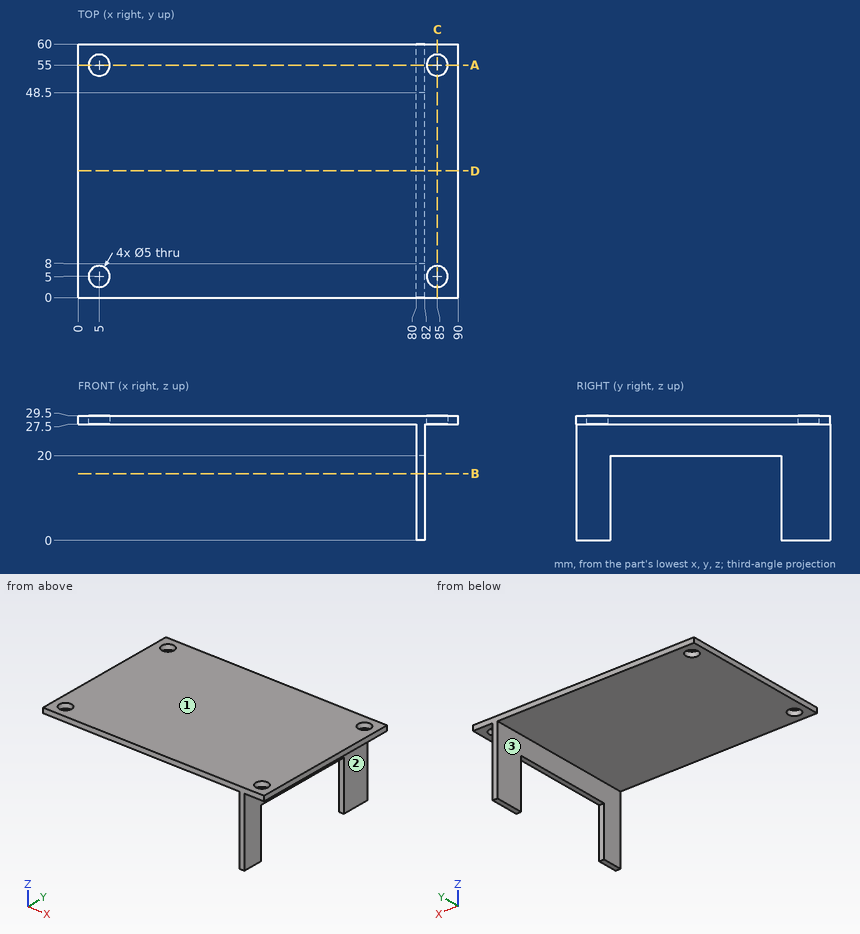
Could you check a few things on this drawing? It's one solid part, dimensions in mm from its lowest x, y, z. A direction names the side the tool comes from. Round coordinates to 2 decimals unless told otherwise and drop trailing zeros. Write each loop counter-clockwise with the first axis right and the second up, starting at its lowest first coordinate (ties: lowest second). Pieces come first, ordered by that corner, then holes. Notation, with made-up numbers: (42, 40) -> (54, 40) arc R17 cw to (54, 68) -> close; hole circle Ø9 at (50.5, -15.75). An arc over 180 degrees is marked (long way). One line per question, with ' | ' between items. Start each with the question number.
1) Suppose I cut it at D-D on y = 30. Write out the boundary of the cut face in (x, z).
2) Suppose I cut it at C-C on x = 85. Write out the boundary of the cut face in (y, z).
3) I need wall thicknesses on line 1 (Y direction, x = 85, z = 28.85); line 2 (Z direction, x = 15, y = 40); line 3 (X direction, y = 7, z = 11.75). Which ranges of each line are inside material? Lowest first, please. Write a range as [from, to].
4) Suppose I cut it at B-B on z = 15.75. Write out the boundary of the cut face in (x, y), then the cut area to 3 significant figures.
5) On a 3-axis mill with a long thin cutter (end or side, diameter ignored), from which of +Z, -Z, +X, -X, +Y, -Y can I reach the whole of each face in a straight line? I mean the marked faces 1, 2 and 3. Say none if no direction works.
6) I'm going to push flat-ended pins straight in: P1, Ø2, axis at x = 43.5, y = 34.5, coming from the -Z side; P2, Ø1.6, axis at x = 80.5, y = 28, coming from the -Z side; P3, Ø3, axis at x = 85, y = 5, coming from the -Z side; P4, Ø10, axis at y = 50, z = 22, coming from the -X side. Where does each tip first touch, or does it pass through?
7) Suppose I cut it at A-A on y = 55. Write out the boundary of the cut face in (x, z).
Return value:
1) outline: (0, 27.5) -> (80, 27.5) -> (80, 20) -> (82, 20) -> (82, 27.5) -> (90, 27.5) -> (90, 29.5) -> (0, 29.5) -> close
2) outline: (0, 27.5) -> (2.5, 27.5) -> (2.5, 29.5) -> (0, 29.5) -> close; (7.5, 27.5) -> (52.5, 27.5) -> (52.5, 29.5) -> (7.5, 29.5) -> close; (57.5, 27.5) -> (60, 27.5) -> (60, 29.5) -> (57.5, 29.5) -> close
3) line 1: y = [0, 2.5], [7.5, 52.5], [57.5, 60] | line 2: z = [27.5, 29.5] | line 3: x = [80, 82]
4) outline: (80, 0) -> (82, 0) -> (82, 8) -> (80, 8) -> close; (80, 48.5) -> (82, 48.5) -> (82, 60) -> (80, 60) -> close | area: 39.0 mm2
5) face 1: +Z, +X, -X, +Y, -Y | face 2: -Z, +X, +Y, -Y | face 3: -Z, -X, +Y, -Y
6) P1: stops at z = 27.5 | P2: stops at z = 20 | P3: passes through | P4: stops at x = 80
7) outline: (0, 27.5) -> (2.5, 27.5) -> (2.5, 29.5) -> (0, 29.5) -> close; (7.5, 27.5) -> (80, 27.5) -> (80, 0) -> (82, 0) -> (82, 27.5) -> (82.5, 27.5) -> (82.5, 29.5) -> (7.5, 29.5) -> close; (87.5, 27.5) -> (90, 27.5) -> (90, 29.5) -> (87.5, 29.5) -> close
